Geometry check sheet. Reference: the model listing, model coordinates, mm. Face numbers are marked on the shaded views. A direction names the side the tool comes from. Round coordinates to 2 decimals unless told otherwise and drop trailing zeros. Order: outer loops, then holes, each group sorted by start corner. A loop starts at its lowest first (then second) coordinate and runs counter-clockwise, first axis right, second up.
(1) Draft check along X on the marked faces 1, 2 and 3. Enter one of: pulls with the +X half, pulls with the -X half, needs draft (parallel to the pull), parting line crosses it, or undercut.
(2) Cross-section at A-A on z = 18.75. Enter the section's corners in (x, y), and give its area (3 significant figures).
(3) Gauge pin test, flat ends, axial feed: P1, Ø12, axis at x = 9.5, y = -12.5, coming from the +Z side; P2, Ø5, axis at y = -12.5, z = 15, coming from the -X side; P3, Ø4, axis at x = 0, y = 0, coming from the +Z side; P4, Ø3, axis at y = 4.5, z = 7.5, coming from the -X side. Record the tip position at first contact, or that the pin passes through.
(4) Cross-section at B-B on y = -3.5. Enter the section's corners in (x, z), and give its area (3 significant figures).
(5) Set-up check for the marked faces 4, 5, 6 and 7: record each of +Z, -Z, +X, -X, +Y, -Y from which the full face is reachable in a straight line by a thin tool's end or side.
(6) Thickness scan on L1, parallel to Y at x = 0, z = 2.75; L2, parallel to Y at x = -20, z = 4; L3, parallel to Z at x = -0.5, y = 18.5. Record the ranges inside material, lowest first.
from build123d import *

# Parameters (mm, degrees)
BOSS_EXTRUDE1_DEPTH = 10.16
SKETCH2_R           = 2.5
CUT_EXTRUDE1_DEPTH  = 10.16
SKETCH5_R           = 2.5
BOSS_EXTRUDE2_DEPTH = 15


with BuildPart() as part:
    # Sketch1 → Boss-Extrude1 (new body)
    with BuildSketch(Plane.XY):
        with BuildLine():
            Line((21.369115072, -12.969065822), (19.986578913, -11.025302977))
            Line((19.986578913, -11.025302977), (17.28565357, -9.025307787))
            ThreePointArc((17.28565357, -9.025307787), (17.644127523, -8.302696186), (17.972409434, -7.565877287))
            Line((17.972409434, -7.565877287), (21.235066822, -8.372131118))
            Line((21.235066822, -8.372131118), (23.614023549, -8.19839247))
            Line((23.614023549, -8.19839247), (23.923040543, -7.247335954))
            Line((23.923040543, -7.247335954), (22.100545137, -5.708462756))
            Line((22.100545137, -5.708462756), (18.987095752, -4.442993911))
            ThreePointArc((18.987095752, -4.442993911), (19.154601389, -3.653935634), (19.289330312, -2.858624865))
            Line((19.289330312, -2.858624865), (22.649992492, -2.828158852))
            Line((22.649992492, -2.828158852), (24.911002874, -2.068256043))
            Line((24.911002874, -2.068256043), (24.973793394, -1.070229315))
            Line((24.973793394, -1.070229315), (22.82585283, -0.032938825))
            Line((22.82585283, -0.032938825), (19.495508879, 0.418489613))
            ThreePointArc((19.495508879, 0.418489613), (19.461521204, 1.224415131), (19.394231625, 2.02824547))
            Line((19.394231625, 2.02824547), (22.641735833, 2.893517036))
            Line((22.641735833, 2.893517036), (24.642732273, 4.191836518))
            Line((24.642732273, 4.191836518), (24.455350958, 5.174123768))
            Line((24.455350958, 5.174123768), (22.116928242, 5.644654774))
            Line((22.116928242, 5.644654774), (18.778947483, 5.253677896))
            ThreePointArc((18.778947483, 5.253677896), (18.545602068, 6.02583139), (18.280522038, 6.787673684))
            Line((18.280522038, 6.787673684), (21.210815641, 8.433382607))
            Line((21.210815641, 8.433382607), (22.826068173, 10.188540573))
            Line((22.826068173, 10.188540573), (22.400288882, 11.093367626))
            Line((22.400288882, 11.093367626), (20.018315712, 10.967573953))
            Line((20.018315712, 10.967573953), (16.882435753, 9.758758274))
            ThreePointArc((16.882435753, 9.758758274), (16.464394547, 10.448622502), (16.01818002, 11.120607396))
            Line((16.01818002, 11.120607396), (18.447141895, 13.443347733))
            Line((18.447141895, 13.443347733), (19.575158262, 15.545061154))
            Line((19.575158262, 15.545061154), (18.937734272, 16.315574397))
            Line((18.937734272, 16.315574397), (16.661878784, 15.601360125))
            Line((16.661878784, 15.601360125), (13.925138495, 13.65065998))
            ThreePointArc((13.925138495, 13.65065998), (13.348668566, 14.214888235), (12.749356841, 14.754792447))
            Line((12.749356841, 14.754792447), (14.524366379, 17.60861788))
            Line((14.524366379, 17.60861788), (15.094269164, 19.924828372))
            Line((15.094269164, 19.924828372), (14.28525217, 20.512613624))
            Line((14.28525217, 20.512613624), (12.258514734, 19.254855463))
            Line((12.258514734, 19.254855463), (10.092873572, 16.684840516))
            ThreePointArc((10.092873572, 16.684840516), (9.394196645, 17.087980261), (8.679444682, 17.461879624))
            Line((8.679444682, 17.461879624), (9.688971507, 20.667473805))
            Line((9.688971507, 20.667473805), (9.664951622, 23.052645345))
            Line((9.664951622, 23.052645345), (8.735175137, 23.420769898))
            Line((8.735175137, 23.420769898), (7.084903119, 21.698497417))
            Line((7.084903119, 21.698497417), (5.626436284, 18.67065116))
            ThreePointArc((5.626436284, 18.67065116), (4.8494528, 18.887371642), (4.064171094, 19.071772684))
            Line((4.064171094, 19.071772684), (4.244782922, 22.427716342))
            Line((4.244782922, 22.427716342), (3.628349625, 24.731979829))
            Line((3.628349625, 24.731979829), (2.636234924, 24.857313063))
            Line((2.636234924, 24.857313063), (1.466120985, 22.778742977))
            Line((1.466120985, 22.778742977), (0.806469312, 19.483316126))
            ThreePointArc((0.806469312, 19.483316126), (0, 19.5), (-0.806469312, 19.483316126))
            Line((-0.806469312, 19.483316126), (-1.466120985, 22.778742977))
            Line((-1.466120985, 22.778742977), (-2.636234924, 24.857313063))
            Line((-2.636234924, 24.857313063), (-3.628349625, 24.731979829))
            Line((-3.628349625, 24.731979829), (-4.244782922, 22.427716342))
            Line((-4.244782922, 22.427716342), (-4.064171094, 19.071772684))
            ThreePointArc((-4.064171094, 19.071772684), (-4.8494528, 18.887371642), (-5.626436284, 18.67065116))
            Line((-5.626436284, 18.67065116), (-7.084903119, 21.698497417))
            Line((-7.084903119, 21.698497417), (-8.735175137, 23.420769898))
            Line((-8.735175137, 23.420769898), (-9.664951622, 23.052645345))
            Line((-9.664951622, 23.052645345), (-9.688971507, 20.667473805))
            Line((-9.688971507, 20.667473805), (-8.679444682, 17.461879624))
            ThreePointArc((-8.679444682, 17.461879624), (-9.394196645, 17.087980261), (-10.092873572, 16.684840516))
            Line((-10.092873572, 16.684840516), (-12.258514734, 19.254855463))
            Line((-12.258514734, 19.254855463), (-14.28525217, 20.512613624))
            Line((-14.28525217, 20.512613624), (-15.094269164, 19.924828372))
            Line((-15.094269164, 19.924828372), (-14.524366379, 17.60861788))
            Line((-14.524366379, 17.60861788), (-12.749356841, 14.754792447))
            ThreePointArc((-12.749356841, 14.754792447), (-13.348668566, 14.214888235), (-13.925138495, 13.65065998))
            Line((-13.925138495, 13.65065998), (-16.661878784, 15.601360125))
            Line((-16.661878784, 15.601360125), (-18.937734272, 16.315574397))
            Line((-18.937734272, 16.315574397), (-19.575158262, 15.545061154))
            Line((-19.575158262, 15.545061154), (-18.447141895, 13.443347733))
            Line((-18.447141895, 13.443347733), (-16.01818002, 11.120607396))
            ThreePointArc((-16.01818002, 11.120607396), (-16.464394547, 10.448622502), (-16.882435753, 9.758758274))
            Line((-16.882435753, 9.758758274), (-20.018315712, 10.967573953))
            Line((-20.018315712, 10.967573953), (-22.400288882, 11.093367626))
            Line((-22.400288882, 11.093367626), (-22.826068173, 10.188540573))
            Line((-22.826068173, 10.188540573), (-21.210815641, 8.433382607))
            Line((-21.210815641, 8.433382607), (-18.280522038, 6.787673684))
            ThreePointArc((-18.280522038, 6.787673684), (-18.545602068, 6.02583139), (-18.778947483, 5.253677896))
            Line((-18.778947483, 5.253677896), (-22.116928242, 5.644654774))
            Line((-22.116928242, 5.644654774), (-24.455350958, 5.174123768))
            Line((-24.455350958, 5.174123768), (-24.642732273, 4.191836518))
            Line((-24.642732273, 4.191836518), (-22.641735833, 2.893517036))
            Line((-22.641735833, 2.893517036), (-19.394231625, 2.02824547))
            ThreePointArc((-19.394231625, 2.02824547), (-19.461521204, 1.224415131), (-19.495508879, 0.418489613))
            Line((-19.495508879, 0.418489613), (-22.82585283, -0.032938825))
            Line((-22.82585283, -0.032938825), (-24.973793394, -1.070229315))
            Line((-24.973793394, -1.070229315), (-24.911002874, -2.068256043))
            Line((-24.911002874, -2.068256043), (-22.649992492, -2.828158852))
            Line((-22.649992492, -2.828158852), (-19.289330312, -2.858624865))
            ThreePointArc((-19.289330312, -2.858624865), (-19.154601389, -3.653935634), (-18.987095752, -4.442993911))
            Line((-18.987095752, -4.442993911), (-22.100545137, -5.708462756))
            Line((-22.100545137, -5.708462756), (-23.923040543, -7.247335954))
            Line((-23.923040543, -7.247335954), (-23.614023549, -8.19839247))
            Line((-23.614023549, -8.19839247), (-21.235066822, -8.372131118))
            Line((-21.235066822, -8.372131118), (-17.972409434, -7.565877287))
            ThreePointArc((-17.972409434, -7.565877287), (-17.644127523, -8.302696186), (-17.28565357, -9.025307787))
            Line((-17.28565357, -9.025307787), (-19.986578913, -11.025302977))
            Line((-19.986578913, -11.025302977), (-21.369115072, -12.969065822))
            Line((-21.369115072, -12.969065822), (-20.833288277, -13.813393747))
            Line((-20.833288277, -13.813393747), (-18.485863806, -13.390051595))
            Line((-18.485863806, -13.390051595), (-15.526215974, -11.797737814))
            ThreePointArc((-15.526215974, -11.797737814), (-15.025008234, -12.4297678), (-14.498090202, -13.040528383))
            Line((-14.498090202, -13.040528383), (-16.61678243, -15.649382865))
            Line((-16.61678243, -15.649382865), (-17.472489512, -17.875901587))
            Line((-17.472489512, -17.875901587), (-16.743520884, -18.560448692))
            Line((-16.743520884, -18.560448692), (-14.575125981, -17.566625886))
            Line((-14.575125981, -17.566625886), (-12.104453263, -15.288303085))
            ThreePointArc((-12.104453263, -15.288303085), (-11.46181242, -15.77583139), (-10.799558506, -16.23636462))
            Line((-10.799558506, -16.23636462), (-12.202892395, -19.290154472))
            Line((-12.202892395, -19.290154472), (-12.478003175, -21.659528712))
            Line((-12.478003175, -21.659528712), (-11.601696495, -22.141282386))
            Line((-11.601696495, -22.141282386), (-9.748579387, -20.639424467))
            Line((-9.748579387, -20.639424467), (-7.922123236, -17.818248046))
            ThreePointArc((-7.922123236, -17.818248046), (-7.178428777, -18.130641475), (-6.422450831, -18.412010355))
            Line((-6.422450831, -18.412010355), (-7.022249752, -21.71885473))
            Line((-7.022249752, -21.71885473), (-6.699478009, -24.08220799))
            Line((-6.699478009, -24.08220799), (-5.730894848, -24.330897877))
            Line((-5.730894848, -24.330897877), (-4.309493697, -22.415372101))
            Line((-4.309493697, -22.415372101), (-3.242017071, -19.228606952))
            ThreePointArc((-3.242017071, -19.228606952), (-2.443998055, -19.346236676), (-1.64179695, -19.430761765))
            Line((-1.64179695, -19.430761765), (-1.40037333, -22.782879469))
            Line((-1.40037333, -22.782879469), (-0.5, -24.991713572))
            Line((-0.5, -24.991713572), (0.5, -24.991713572))
            Line((0.5, -24.991713572), (1.40037333, -22.782879469))
            Line((1.40037333, -22.782879469), (1.64179695, -19.430761765))
            ThreePointArc((1.64179695, -19.430761765), (2.443998055, -19.346236676), (3.242017071, -19.228606952))
            Line((3.242017071, -19.228606952), (4.309493697, -22.415372101))
            Line((4.309493697, -22.415372101), (5.730894848, -24.330897877))
            Line((5.730894848, -24.330897877), (6.699478009, -24.08220799))
            Line((6.699478009, -24.08220799), (7.022249752, -21.71885473))
            Line((7.022249752, -21.71885473), (6.422450831, -18.412010355))
            ThreePointArc((6.422450831, -18.412010355), (7.178428777, -18.130641475), (7.922123236, -17.818248046))
            Line((7.922123236, -17.818248046), (9.748579387, -20.639424467))
            Line((9.748579387, -20.639424467), (11.601696495, -22.141282386))
            Line((11.601696495, -22.141282386), (12.478003175, -21.659528712))
            Line((12.478003175, -21.659528712), (12.202892395, -19.290154472))
            Line((12.202892395, -19.290154472), (10.799558506, -16.23636462))
            ThreePointArc((10.799558506, -16.23636462), (11.46181242, -15.77583139), (12.104453263, -15.288303085))
            Line((12.104453263, -15.288303085), (14.575125981, -17.566625886))
            Line((14.575125981, -17.566625886), (16.743520884, -18.560448692))
            Line((16.743520884, -18.560448692), (17.472489512, -17.875901587))
            Line((17.472489512, -17.875901587), (16.61678243, -15.649382865))
            Line((16.61678243, -15.649382865), (14.498090202, -13.040528383))
            ThreePointArc((14.498090202, -13.040528383), (15.025008234, -12.4297678), (15.526215974, -11.797737814))
            Line((15.526215974, -11.797737814), (18.485863806, -13.390051595))
            Line((18.485863806, -13.390051595), (20.833288277, -13.813393747))
            Line((20.833288277, -13.813393747), (21.369115072, -12.969065822))
        make_face()
    extrude(amount=BOSS_EXTRUDE1_DEPTH)

    # Sketch2 → Cut-Extrude1 (cut)
    with BuildSketch(Plane.XY.offset(10.16)):
        Circle(SKETCH2_R)
    extrude(amount=-CUT_EXTRUDE1_DEPTH, mode=Mode.SUBTRACT)

    # Sketch5 → Boss-Extrude2 (add)
    with BuildSketch(Plane.XY.offset(10.16)):
        with Locations((0, -13.406225592)):
            Circle(SKETCH5_R)
    extrude(amount=BOSS_EXTRUDE2_DEPTH)


solid = part.part
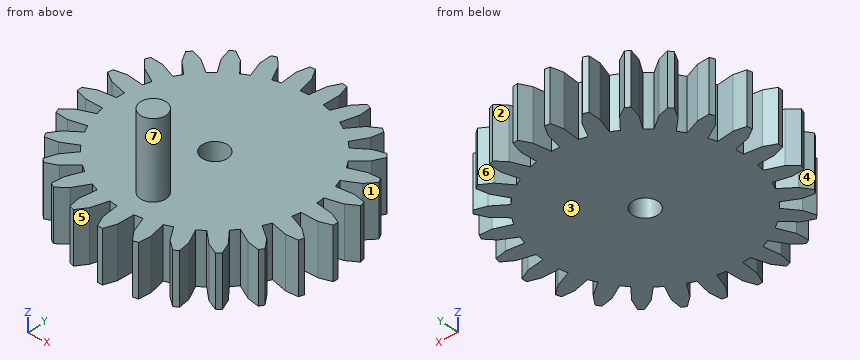
Found:
1. face 1: pulls with the +X half
1. face 2: undercut
1. face 3: needs draft
2. outline: circle Ø5 at (0, -13.41)
2. area: 19.6 mm2
3. P1: stops at z = 10.16
3. P2: stops at x = -2.5
3. P3: passes through
3. P4: stops at x = -24.64
4. outline: (-19.18, 0) - (19.18, 0) - (19.18, 10.16) - (-19.18, 10.16) - close
4. area: 390 mm2
5. face 4: +Z, -Z, -X
5. face 5: +Z, -Z, -Y
5. face 6: +Z, -Z, +Y
5. face 7: +Z
6. L1: y = -24.99 to -2.5, 2.5 to 19.5
6. L2: y = -13.66 to -11.04, -8.07 to -4.85, -2.85 to 0.35, 2.19 to 5.4, 7.75 to 10.96
6. L3: z = 0 to 10.16
